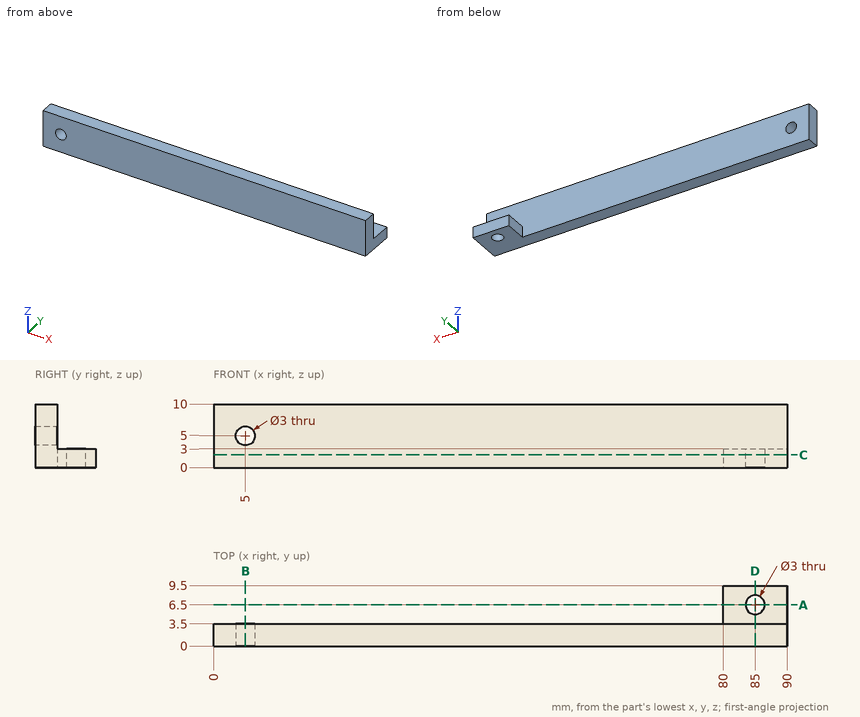
Design review of the part shown in the three views and the two pictorial views. Dimensions are in mm from the part's minimum x, y and z. Round coordinates to 2 decimals unless told otherwise and drop trailing zeros. Write each loop counter-clockwise with the first axis right and the second up, starting at its lowest first coordinate (ties: lowest second). Pieces come first, ordered by that corner, then holes. Notation, with made-up numbers: (83, -20) - (132, -20) arc R35 cw to (132, 16) - close; hole circle Ø9 at (-4.5, 41.25). An arc over 180 degrees is marked (long way). Return JSON: item names as keys, results as strings. Group by question number.
Item 1: We need section B-B on x = 5. Write out the cut boundary in (y, z), and give its area (3 significant figures).
Item 2: Insertion check: P1, Ø3, axis at x = 44.5, y = 6.5, coming from the -Z side; P2, Ø3, axis at x = 57.5, z = 4, coming from the +Y side; P3, Ø0.9, axis at y = 6.5, z = 1, coming from the -X side. Each pin has a flat end and moves straight along its axis. Give the tip position at first contact, or say it passes through.
Item 3: For probe 1 along X at (y, z) = (2.4, 5); probe 2 along Y at (x, z) = (85, 1.4); probe 3 along Y at (x, z) = (39.5, 5), list the stretches that pass through material, from the lowest coordinate up. Write a range as [from, to].
Item 4: We need section C-C on z = 2. Write out the cut boundary in (x, y).
Item 5: We need section A-A on y = 6.5. Write out the cut boundary in (x, z).
Item 6: We need section D-D on x = 85. Write out the cut boundary in (y, z), and give its area (3 significant figures).
Model answer:
{
 "1": {"outline": "(0, 0) - (3.5, 0) - (3.5, 3.5) - (0, 3.5) - close; (0, 6.5) - (3.5, 6.5) - (3.5, 10) - (0, 10) - close", "area": "24.5 mm²"},
 "2": {"P1": "passes through", "P2": "stops at y = 3.5", "P3": "stops at x = 80"},
 "3": {"probe 1": "x = [0, 3.5], [6.5, 90]", "probe 2": "y = [0, 5], [8, 9.5]", "probe 3": "y = [0, 3.5]"},
 "4": {"outline": "(0, 0) - (90, 0) - (90, 9.5) - (80, 9.5) - (80, 3.5) - (0, 3.5) - close; hole circle Ø3 at (85, 6.5)"},
 "5": {"outline": "(80, 0) - (83.5, 0) - (83.5, 3) - (80, 3) - close; (86.5, 0) - (90, 0) - (90, 3) - (86.5, 3) - close"},
 "6": {"outline": "(0, 0) - (5, 0) - (5, 3) - (3.5, 3) - (3.5, 10) - (0, 10) - close; (8, 0) - (9.5, 0) - (9.5, 3) - (8, 3) - close", "area": "44.0 mm²"}
}
